Check sheet for the modelled part. Datum: model origin and axes. Units: mm. Face numbers are marked on the shaded views. A direction names the side the tool comes from. Coordinates: 2 decimals unless noted, no trailing zeros. Loops run counter-clockwise (first coordinate to the right, second up) from the corner with the lowest first, then second, coordinate; pieces in that order, holes last. Notation, with made-up numbers: M 85,46.25 L 109,46.25 A15 cw 109,72.25 Z; hole C -17,-3 d9. An arc over 180 degrees is marked long. Return JSON: item names as keys, results as strings.
from build123d import *

# Parameters (mm, degrees)
F1_DEPTH = 6.35
F3_DEPTH = 6.35


with BuildPart() as f1:
    # F0 (on Top) → F1 (new body)
    with BuildSketch(Plane.XY):
        Polygon((11.083248, 37.27174), (-13.177601, 37.27174), (-13.177601, 30.92174), (-19.527601, 30.92174), (-19.527601, 24.57174), (-25.877601, 24.57174), (-25.877601, -26.22826), (-19.527601, -26.22826), (-19.527601, -32.57826), (-13.177601, -32.57826), (-13.177601, -38.92826), (11.083248, -38.92826), (11.083248, -32.57826), (17.433248, -32.57826), (17.433248, -26.22826), (23.783248, -26.22826), (23.783248, 24.57174), (17.433248, 24.57174), (17.433248, 30.92174), (11.083248, 30.92174), align=None)
    extrude(amount=F1_DEPTH)

    # F2 (on face) → F3 (join)
    with BuildSketch(Plane.XY.offset(6.35)):
        Polygon((11.083248, 30.92174), (-13.177601, 30.92174), (-13.177601, 24.57174), (-19.527601, 24.57174), (-19.527601, -26.22826), (-13.177601, -26.22826), (-13.177601, -32.57826), (11.083248, -32.57826), (11.083248, -26.22826), (17.433248, -26.22826), (17.433248, 24.57174), (11.083248, 24.57174), align=None)
    extrude(amount=F3_DEPTH)


solid = f1.part
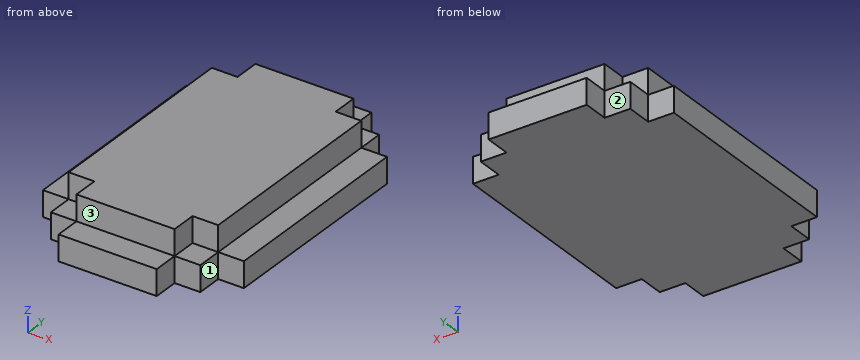
1) Section check D-D on z = 2.75. Record the cut outline in (x, y).
Answers:
{"outline": "M -25.88,-26.23 L -19.53,-26.23 L -19.53,-32.58 L -13.18,-32.58 L -13.18,-38.93 L 11.08,-38.93 L 11.08,-32.58 L 17.43,-32.58 L 17.43,-26.23 L 23.78,-26.23 L 23.78,24.57 L 17.43,24.57 L 17.43,30.92 L 11.08,30.92 L 11.08,37.27 L -13.18,37.27 L -13.18,30.92 L -19.53,30.92 L -19.53,24.57 L -25.88,24.57 Z"}
2) Section check C-C on y = 0.5. Record the cut outline in (x, z), then the cut area to 3 significant figures.
Answers:
{"outline": "M -25.88,0 L 23.78,0 L 23.78,6.35 L 17.43,6.35 L 17.43,12.7 L -19.53,12.7 L -19.53,6.35 L -25.88,6.35 Z", "area": "550 mm²"}
3) Section check A-A on x = -5. Record the cut outline in (y, z), then the cut area to 3 significant figures.
Answers:
{"outline": "M -38.93,0 L 37.27,0 L 37.27,6.35 L 30.92,6.35 L 30.92,12.7 L -32.58,12.7 L -32.58,6.35 L -38.93,6.35 Z", "area": "887 mm²"}
4) Set-up check for the marked faces 1, 2 and 3: record each of +Z, -Z, +X, -X, +Y, -Y from which the full face is reachable in a straight line by a thin tool's end or side.
Answers:
{"face 1": "+Z, -Z, +X, -Y", "face 2": "+Z, -Z, -X, +Y", "face 3": "+Z, +X, -X, -Y"}
5) Section check B-B on z = 7.25. Record the cut outline in (x, y).
Answers:
{"outline": "M -19.53,-26.23 L -13.18,-26.23 L -13.18,-32.58 L 11.08,-32.58 L 11.08,-26.23 L 17.43,-26.23 L 17.43,24.57 L 11.08,24.57 L 11.08,30.92 L -13.18,30.92 L -13.18,24.57 L -19.53,24.57 Z"}
6) Go/stop test with flat-tipped pins: pin 1 Ø3 at (x, y) = (-17, 28) entering from +Z; pin 2 Ø4 at (x, z) = (10, 8.5) entering from +Y; pin 3 Ø5 at (y, z) = (28, 9.5) entering from -X. Record where each tip stops, or that it passes through.
Answers:
{"pin 1": "z = 6.35", "pin 2": "y = 30.92", "pin 3": "x = -13.18"}
7) Scan lines: line 1 along Z through (x, y) = (1, 32); line 2 along Y through (x, z) = (16.5, 2.5); line 3 along X through (y, z) = (-19, 9.5). Record each from-to range of solid material in increasing order. Write a range as [from, to].
Answers:
{"line 1": "[0, 6.35]", "line 2": "[-32.58, 30.92]", "line 3": "[-19.53, 17.43]"}
